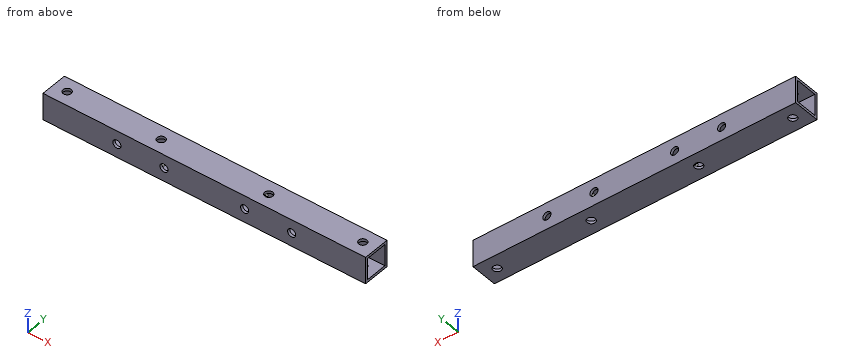
from build123d import *

# Parameters (mm, degrees)
SKETCH_1_W          = 10
SKETCH_1_H          = 10
SKETCH_1_W_2        = 8
SKETCH_1_H_2        = 8
EXTRUDE_1_DEPTH     = 120
SKETCH_2_R          = 1.5
CUT_EXTRUDE_1_DEPTH = 121.519707932
SKETCH_3_R          = 1.5
CUT_EXTRUDE_2_DEPTH = 121.519707932


with BuildPart() as part:
    # ｽｹｯﾁ1 → 押し出し-薄板1 (new body)
    with BuildSketch(Plane(origin=(0, 0, 0), x_dir=(0, 0, -1), z_dir=(1, 0, 0))):
        Rectangle(SKETCH_1_W, SKETCH_1_H)
        Rectangle(SKETCH_1_W_2, SKETCH_1_H_2, mode=Mode.SUBTRACT)
    extrude(amount=EXTRUDE_1_DEPTH)

    # ｽｹｯﾁ2 → ｶｯﾄ - 押し出し1 (cut, through all)
    with BuildSketch(Plane.XY.offset(5)):
        with Locations((5, 0)):
            Circle(SKETCH_2_R)
        with Locations(Location((115, 0, 0), (0, 0, 180))):
            Circle(SKETCH_2_R)
        with Locations((40, 0)):
            Circle(SKETCH_2_R)
        with Locations(Location((80, 0, 0), (0, 0, 180))):
            Circle(SKETCH_2_R)
    extrude(amount=-CUT_EXTRUDE_1_DEPTH, mode=Mode.SUBTRACT)

    # ｽｹｯﾁ3 → ｶｯﾄ - 押し出し2 (cut, through all)
    with BuildSketch(Plane(origin=(0, 5, 0), x_dir=(1, 0, 0), z_dir=(0, 1, 0))):
        with Locations(Location((45, 0, 0), (0, 0, 270))):
            Circle(SKETCH_3_R)
        with Locations(Location((75, 0, 0), (0, 0, 270))):
            Circle(SKETCH_3_R)
        with Locations(Location((27.5, 0, 0), (0, 0, 270))):
            Circle(SKETCH_3_R)
        with Locations(Location((92.5, 0, 0), (0, 0, 270))):
            Circle(SKETCH_3_R)
    extrude(amount=-CUT_EXTRUDE_2_DEPTH, mode=Mode.SUBTRACT)


solid = part.part
CAD build for the part. Positions are in the model's coordinates, mm. Coordinates: 2 decimals unless noted, no trailing zeros. Loops run counter-clockwise (first coordinate to the right, second up) from the corner with the lowest first, then second, coordinate; pieces in that order, holes last. Notation, with made-up numbers: (69.25, -18) -> (84.25, -18) arc R17 cw to (84.25, -14) -> close; hole circle Ø5 at (-34.75, 73.5). An arc over 180 degrees is marked (long way). One line per item, written item: value.
1. Drill centre lines: line 1 (X direction, y = 4.8, z = 0); line 2 (Y direction, x = 9, z = 3.25). Where is each one in solid material? Low to high. Write a range as [from, to].
Answers:
line 1: x = [0, 26], [29, 43.5], [46.5, 73.5], [76.5, 91], [94, 120]
line 2: y = [-5, -4], [4, 5]
2. Slice it at A-A on x = 92.5. Write the cut outline in (y, z), and give its area (3 significant figures).
Answers:
outline: (-5, -5) -> (5, -5) -> (5, -1.5) -> (4, -1.5) -> (4, -4) -> (-4, -4) -> (-4, -1.5) -> (-5, -1.5) -> close; (-5, 1.5) -> (-4, 1.5) -> (-4, 4) -> (4, 4) -> (4, 1.5) -> (5, 1.5) -> (5, 5) -> (-5, 5) -> close
area: 30.0 mm^2
3. Slice it at B-B on z = 2.75. Write the cut outline in (x, y), and give its area (3 significant figures).
Answers:
outline: (0, -5) -> (120, -5) -> (120, -4) -> (0, -4) -> close; (0, 4) -> (120, 4) -> (120, 5) -> (0, 5) -> close
area: 240 mm^2
4. Slice it at C-C on x = 60. Write the cut outline in (y, z).
Answers:
outline: (-5, -5) -> (5, -5) -> (5, 5) -> (-5, 5) -> close; hole (-4, -4) -> (4, -4) -> (4, 4) -> (-4, 4) -> close
5. Slice it at D-D on y = 0. Give the number of separate pieces and of enclosed holes in the cut face, and give its area (3 significant figures).
Answers:
separate pieces: 10
enclosed holes: 0
area: 216 mm^2
